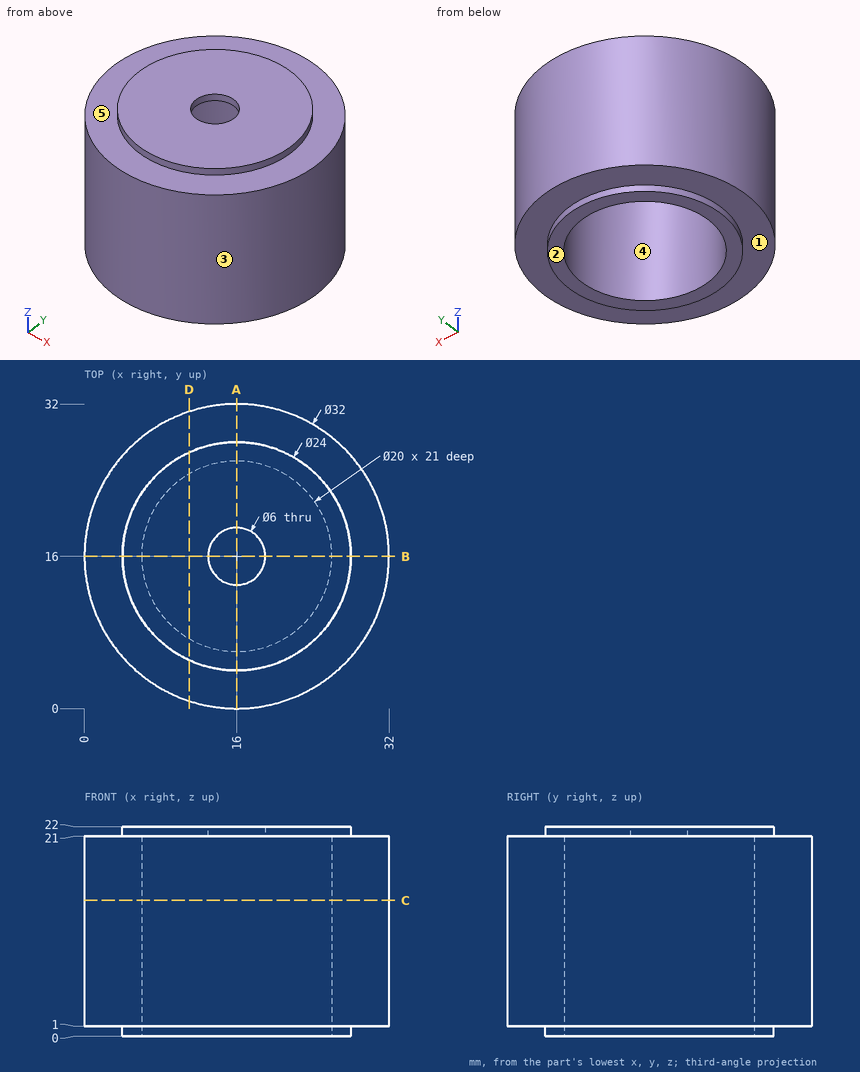
Design review of the part shown in the three views and the two pictorial views. Dimensions are in mm from the part's minimum x, y and z. A direction names the side the tool comes from. Round coordinates to 2 decimals unless told otherwise and drop trailing zeros. Order: outer loops, then holes, each group sorted by start corner. A loop starts at its lowest first (then second) coordinate and runs counter-clockwise, first axis right, second up. Notation, with made-up numbers: M 45,65 L 88,65 A12 ccw 88,74 Z; hole C 52.25,43 d9. An arc over 180 degrees is marked long. Put each result on its own line as item: value.
Q1. Consider section D-D (x = 11). State the section outline as (y, z) points.
Reported:
outline: M 0.8,1 L 5.09,1 L 5.09,0 L 7.34,0 L 7.34,21 L 24.66,21 L 24.66,0 L 26.91,0 L 26.91,1 L 31.2,1 L 31.2,21 L 26.91,21 L 26.91,22 L 5.09,22 L 5.09,21 L 0.8,21 Z
Q2. Draft analysis for pull direction X (two halves, no side actions). For the marked faces 3, 4 and 5, state which applies: released by +X, released by -X, zero draft, split by the parting line, or undercut.
Reported:
face 3: split by the parting line
face 4: undercut
face 5: zero draft
Q3. To check wall thickness, follow line 1 (Y direction, x = 16, z = 7); line 2 (Z direction, x = 3.5, y = 12.5); line 3 (Z direction, x = 19, y = 8.5). State the ranges of each line that lie inside material, in increasing order.
Reported:
line 1: 0 to 6, 26 to 32
line 2: 1 to 21
line 3: 21 to 22
Q4. Consider section C-C (z = 14.25). State the section outline as (x, y) points, and give its area (3 significant figures).
Reported:
outline: C 16,16 d32; hole C 16,16 d20
area: 490 mm²
Q5. Insertion check: pin 1 Ø1 at (y, z) = (26.5, 16) entering from +X; pin 2 Ø1 at (x, z) = (12, 3) entering from +Y; pin 3 Ø9.5 at (x, y) = (18.5, 12.5) entering from -Z. Each pin has a flat end and moves straight along its axis. Give the tip position at first contact, or say it passes through.
Reported:
pin 1: x = 28.49
pin 2: y = 31.61
pin 3: z = 21
Q6. Machinability: for the marked faces 1 and 2, which of the approach directions +Z, -Z, +X, -X, +Y, -Y give a long, thin tool a straight path to every point of the face, cutting with its end or side? Answer none if there is none.
Reported:
face 1: -Z
face 2: -Z, +X, -X, +Y, -Y
Q7. Consider section A-A (x = 16). State the section outline as (y, z) points, and give its area (3 significant figures).
Reported:
outline: M 0,1 L 4,1 L 4,0 L 6,0 L 6,21 L 13,21 L 13,22 L 4,22 L 4,21 L 0,21 Z; M 19,21 L 26,21 L 26,0 L 28,0 L 28,1 L 32,1 L 32,21 L 28,21 L 28,22 L 19,22 Z
area: 262 mm²
